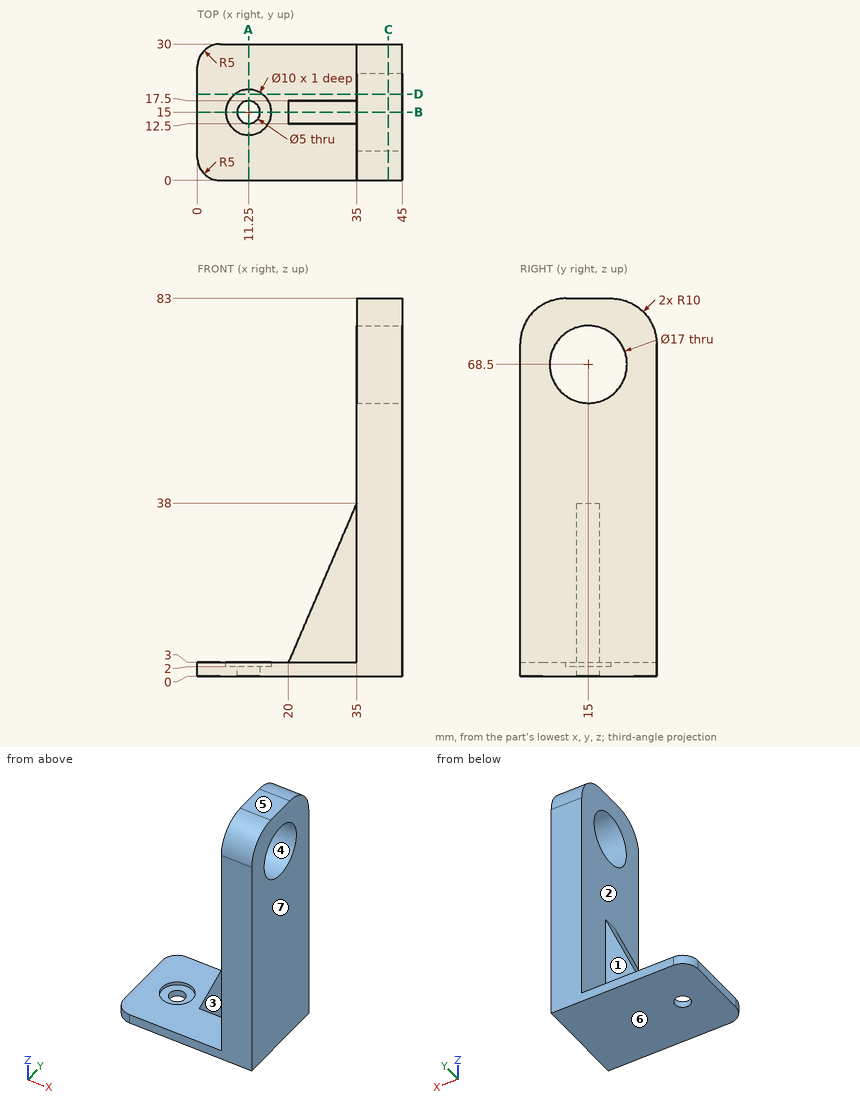
For this review, use the dimensioned drawing (mm, ordinates from the lowest corner) and the shaded views. A direction names the side the tool comes from. Coordinates: 2 decimals unless noted, no trailing zeros. Write each loop counter-clockwise with the first axis right and the second up, starting at its lowest first coordinate (ties: lowest second). Pieces come first, ordered by that corner, then holes. Notation, with made-up numbers: (22.25, -13) -> (27.25, -13) arc R19 cw to (27.25, -1) -> close; hole circle Ø4 at (59.25, 8.25). An arc over 180 degrees is marked (long way). Write each question's results on one line, items separated by ' | '. Start each with the question number.
(1) Take a section at B-B on y = 15. Write out the cut boundary in (x, z).
(2) For line 1 along Y through (x, z) = (41, 68); line 2 along Y through (x, z) = (24, 10.5); line 3 along Z through (x, y) = (34, 8.5), list the stretches that pass through material, from the lowest coordinate up. Write a range as from..to.
(3) Take a section at A-A on x = 11.25. Write out the cut boundary in (y, z).
(4) Take a section at D-D on y = 19. Write out the cut boundary in (x, z), and give its area (3 significant figures).
(5) Clearance check with flat-ended pins moving along their axes: P1, Ø8, axis at x = 17, y = 13.5, coming from the +Z side; P2, Ø12, axis at x = 26.5, z = 17.5, coming from the -Y side; P3, Ø9, axis at x = 18, y = 22, coming from the +Z side; P4, Ø10, axis at x = 26, z = 43, coming from the -Y side. State where each tip first meets the part, or that it passes through.
(6) The part is to be moulded in two halves that separate along Z. For the marked faces 4, 5, 6 and 7, say which applies: pulls with the +Z half, pulls with the -Z half, needs draft (parallel to the pull), parting line crosses it, or undercut.
(7) Tool access review of the marked faces 1, 2 and 3: name each direction out of +Z, -Z, +X, -X, +Y, -Y from which nothing blocks a thin tool from reaching the whole face with its end or side.
(8) Take a section at C-C on x = 42. Write out the cut boundary in (y, z).
Results found:
1) outline: (0, 0) -> (8.75, 0) -> (8.75, 2) -> (6.25, 2) -> (6.25, 3) -> (0, 3) -> close; (13.75, 0) -> (45, 0) -> (45, 60) -> (35, 60) -> (35, 38) -> (20, 3) -> (16.25, 3) -> (16.25, 2) -> (13.75, 2) -> close; (35, 77) -> (45, 77) -> (45, 83) -> (35, 83) -> close
2) line 1: y = 0..6.51, 23.49..30 | line 2: y = 12.5..17.5 | line 3: z = 0..3
3) outline: (0, 0) -> (12.5, 0) -> (12.5, 2) -> (10, 2) -> (10, 3) -> (0, 3) -> close; (17.5, 0) -> (30, 0) -> (30, 3) -> (20, 3) -> (20, 2) -> (17.5, 2) -> close
4) outline: (0, 0) -> (45, 0) -> (45, 61) -> (35, 61) -> (35, 3) -> (14.25, 3) -> (14.25, 2) -> (8.25, 2) -> (8.25, 3) -> (0, 3) -> close; (35, 76) -> (45, 76) -> (45, 83) -> (35, 83) -> close | area: 779 mm2
5) P1: stops at z = 5.33 | P2: stops at y = 12.5 | P3: stops at z = 3 | P4: passes through
6) face 4: undercut | face 5: pulls with the +Z half | face 6: pulls with the -Z half | face 7: needs draft
7) face 1: +Z, -X, +Y | face 2: +Z, -X | face 3: +Z, -X, -Y
8) outline: (0, 0) -> (30, 0) -> (30, 73) arc R10 ccw to (20, 83) -> (10, 83) arc R10 ccw to (0, 73) -> close; hole circle Ø17 at (15, 68.5)
